Can you work these out from the drawing? Everything is in mm from the part's minimum corner. Round coordinates to 2 decimals unless told otherwise and drop trailing zeros. Write each loop counter-clockwise with the first axis right and the second up, starting at its lowest first coordinate (ties: lowest second). Pieces come first, ordered by that corner, then holes.
Q1. If we section it at B-B (y = 15): Please give me the cut outline in (x, z), plus the area to 3 significant figures.
Q2. If we section it at A-A (x = 31): Please give me the cut outline in (y, z), plus the area to 3 significant figures.
Q3. I'm going to push a flat-ended pin straight in: pin 1 Ø3.5 at (x, y) = (56, 15) entering from -Z. Where does the tip first touch, or does it pass through?
Q4. If we section it at C-C (x = 24): Please give me the cut outline in (y, z).
Q5. Please list where these lines run through material, in increasing order: line 1 along Y through (x, z) = (31, 6.15); line 2 along X through (y, z) = (14, 3.25); line 3 along Y through (x, z) = (56, 5).
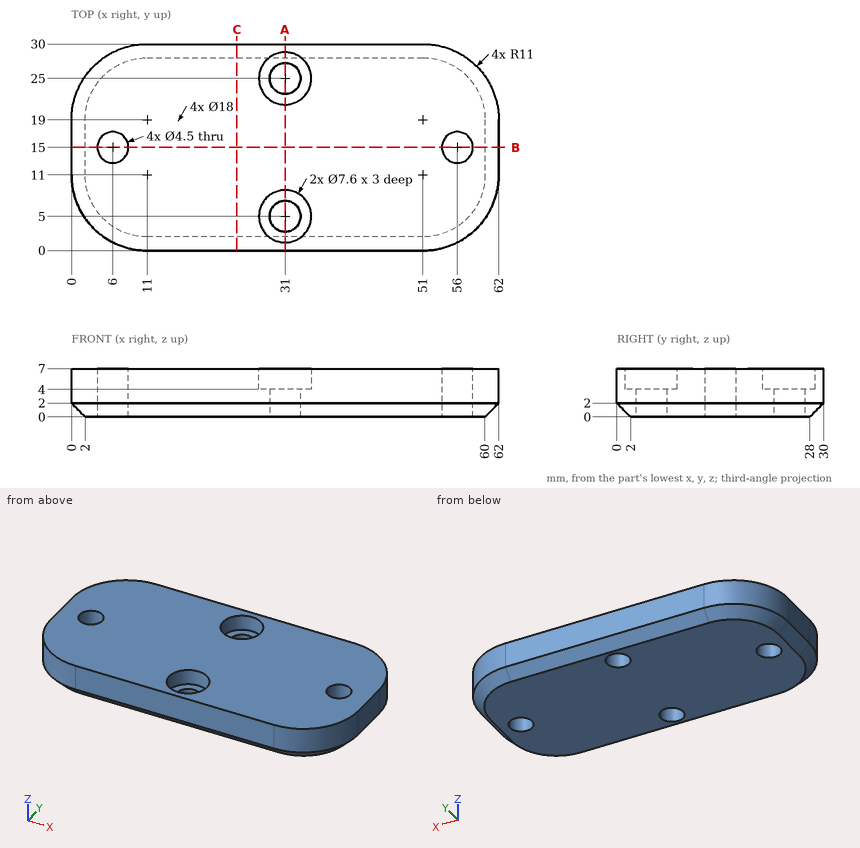
A:
1. outline: (0, 2) - (2, 0) - (3.75, 0) - (3.75, 7) - (0, 7) - close; (8.25, 0) - (53.75, 0) - (53.75, 7) - (8.25, 7) - close; (58.25, 0) - (60, 0) - (62, 2) - (62, 7) - (58.25, 7) - close
1. area: 367 mm2
2. outline: (0, 2) - (2, 0) - (2.75, 0) - (2.75, 4) - (1.2, 4) - (1.2, 7) - (0, 7) - close; (7.25, 0) - (22.75, 0) - (22.75, 4) - (21.2, 4) - (21.2, 7) - (8.8, 7) - (8.8, 4) - (7.25, 4) - close; (27.25, 0) - (28, 0) - (30, 2) - (30, 7) - (28.8, 7) - (28.8, 4) - (27.25, 4) - close
2. area: 124 mm2
3. pin 1: passes through
4. outline: (0, 2) - (2, 0) - (28, 0) - (30, 2) - (30, 7) - (0, 7) - close
5. line 1: y = 0 to 1.2, 8.8 to 21.2, 28.8 to 30
5. line 2: x = 0 to 3.98, 8.02 to 53.98, 58.02 to 62
5. line 3: y = 1.2 to 12.75, 17.25 to 28.8
